Design review of the part shown in the three views and the two pictorial views. Dimensions are in mm from the part's minimum x, y and z. Give positions to 0.01 mm unless a question says otherwise; leave off trailing zeros. Order: outer loops, then holes, each group sorted by start corner. A loop starts at its lowest first (then second) coordinate and runs counter-clockwise, first axis right, second up. Notation, with made-up numbers: M 12,15 L 51,15 A22 cw 51,31 Z; hole C 85.25,-35 d8. An arc over 180 degrees is marked long. Answer as a JSON object with one key per item and string values.
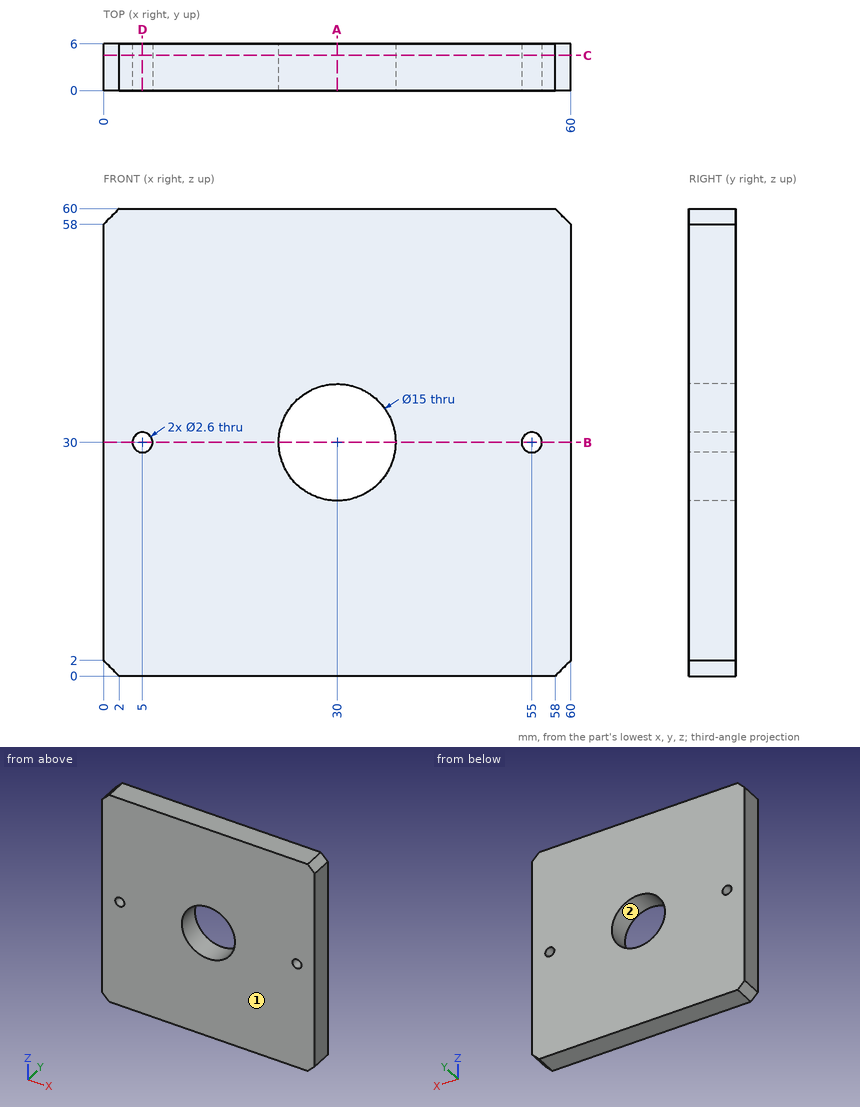
(1) We need section D-D (x = 5). Write out the cut boundary in (y, z).
Checked values:
{"outline": "M 0,0 L 6,0 L 6,28.7 L 0,28.7 Z; M 0,31.3 L 6,31.3 L 6,60 L 0,60 Z"}
(2) We need section A-A (x = 30). Write out the cut boundary in (y, z).
Checked values:
{"outline": "M 0,0 L 6,0 L 6,22.5 L 0,22.5 Z; M 0,37.5 L 6,37.5 L 6,60 L 0,60 Z"}
(3) To check wall thickness, follow L1, parallel to Z at x = 30, y = 3.7; L2, parallel to Z at x = 5, y = 4.55. State the ranges of each line that lie inside material, in increasing order. Write a range as from..to.
Checked values:
{"L1": "z = 0..22.5, 37.5..60", "L2": "z = 0..28.7, 31.3..60"}
(4) Draft analysis for pull direction X (two halves, no side actions). For the marked faces 1 and 2, state which applies: +X half, -X half, draft (parallel to the pull), parting line (faces both ways), or undercut.
Checked values:
{"face 1": "draft", "face 2": "undercut"}
(5) We need section C-C (y = 4.55). Write out the cut boundary in (x, z).
Checked values:
{"outline": "M 0,2 L 2,0 L 58,0 L 60,2 L 60,58 L 58,60 L 2,60 L 0,58 Z; hole C 5,30 d2.6; hole C 30,30 d15; hole C 55,30 d2.6"}
(6) We need section B-B (z = 30). Write out the cut boundary in (x, y), plus the area to 3 significant figures.
Checked values:
{"outline": "M 0,0 L 3.7,0 L 3.7,6 L 0,6 Z; M 6.3,0 L 22.5,0 L 22.5,6 L 6.3,6 Z; M 37.5,0 L 53.7,0 L 53.7,6 L 37.5,6 Z; M 56.3,0 L 60,0 L 60,6 L 56.3,6 Z", "area": "239 mm^2"}
